Read the model definition and answer for the solid it produces. Units are mm, in the model's axes. A direction names the side the tool comes from. Coordinates: 2 decimals unless noted, no trailing zeros. Order: outer loops, then holes, each group sorted by start corner. A loop starts at its lowest first (then second) coordinate and runs counter-clockwise, first axis right, second up.
from build123d import *

# Parameters (mm, degrees)
SKETCH1_W           = 34
SKETCH1_H           = 29
SKETCH1_R           = 1.4
SKETCH1_R_2         = 1.5
BOSS_EXTRUDE1_DEPTH = 5
BOSS_EXTRUDE2_DEPTH = 5
SKETCH3_R           = 0.85
BOSS_EXTRUDE3_DEPTH = 7
CUT_EXTRUDE2_DEPTH  = 5
FILLET1_R           = 4
SKETCH7_W           = 5
SKETCH7_H           = 34
CUT_EXTRUDE3_DEPTH  = 44
SKETCH8_R           = 1.95
CUT_EXTRUDE4_DEPTH  = 6
FILLET2_R           = 10
BOSS_EXTRUDE4_DEPTH = 4.5
CUT_EXTRUDE5_START  = 4.5
SKETCH9_R           = 2
CUT_EXTRUDE5_DEPTH  = 5
FILLET3_R           = 2


with BuildPart() as part:
    # Sketch1 → Boss-Extrude1 (new body)
    with BuildSketch(Plane.XY):
        with Locations((7.610207842, -10)):
            Rectangle(SKETCH1_W, SKETCH1_H)
        with Locations((15.010207842, 0)):
            Circle(SKETCH1_R, mode=Mode.SUBTRACT)
        with Locations((15.010207842, -20)):
            Circle(SKETCH1_R, mode=Mode.SUBTRACT)
        with Locations((0.010207842, 0)):
            Circle(SKETCH1_R_2, mode=Mode.SUBTRACT)
        with Locations((0.010207842, -20)):
            Circle(SKETCH1_R_2, mode=Mode.SUBTRACT)
    extrude(amount=BOSS_EXTRUDE1_DEPTH)

    # Sketch2 → Boss-Extrude2 (add)
    with BuildSketch(Plane.XZ.offset(24.5)):
        Polygon((-9.389792158, -10), (-9.389792158, 5), (24.610207842, 5), (24.610207842, -48), (14.610207842, -48), align=None)
    extrude(amount=BOSS_EXTRUDE2_DEPTH)

    # Sketch3 → Boss-Extrude3 (add)
    with BuildSketch(Plane(origin=(0, -24.5, 0), x_dir=(1, 0, 0), z_dir=(0, 1, 0))):
        Polygon((24.610207842, 40.5), (9.873365737, 40.5), (13.031260474, 45.5), (24.610207842, 45.5), align=None)
        with Locations(Location((18.031260474, 43, 0), (0, 0, 270))):  # turned: the seam where the file's is
            Circle(SKETCH3_R, mode=Mode.SUBTRACT)
    extrude(amount=BOSS_EXTRUDE3_DEPTH)

    # Sketch6 → Cut-Extrude2 (cut)
    with BuildSketch(Plane(origin=(0, -24.5, 0), x_dir=(1, 0, 0), z_dir=(0, 1, 0))):
        Polygon((13.031260474, 45.5), (24.610207842, 45.5), (24.610207842, 48), (14.610207842, 48), align=None)
    extrude(amount=-CUT_EXTRUDE2_DEPTH, mode=Mode.SUBTRACT)

    # Fillet1
    fillet1_edges = [part.edges().sort_by_distance(p)[0] for p in [
        (17.24178679, -24.5, -40.5),
    ]]
    fillet(fillet1_edges, radius=FILLET1_R)

    # Sketch7 → Cut-Extrude3 (cut)
    with BuildSketch(Plane.ZY.offset(9.389792158)):
        with Locations((2.5, -12.5)):
            Rectangle(SKETCH7_W, SKETCH7_H)
    extrude(amount=-CUT_EXTRUDE3_DEPTH, mode=Mode.SUBTRACT)

    # Sketch8 → Cut-Extrude4 (cut)
    with BuildSketch(Plane.XY):
        with Locations((15.110207842, -27)):
            Circle(SKETCH8_R)
        with Locations(Location((0.110207842, -27, 0), (0, 0, 180))):  # turned: the seam where the file's is
            Circle(SKETCH8_R)
    extrude(amount=-CUT_EXTRUDE4_DEPTH, mode=Mode.SUBTRACT)

    # Fillet2
    fillet2_edges = [part.edges().sort_by_distance(p)[0] for p in [
        (-9.389792158, -27, -10),
    ]]
    fillet(fillet2_edges, radius=FILLET2_R)

    # Sketch11 → Boss-Extrude4 (add)
    with BuildSketch(Plane(origin=(0, -24.5, 0), x_dir=(1, 0, 0), z_dir=(0, 1, 0))):
        with BuildLine():
            Line((1.473365737, 27.2), (4.332633033, 27.2))
            ThreePointArc((4.332633033, 27.2), (5.746846596, 26.614213562), (6.332633033, 25.2))
            Line((6.332633033, 25.2), (6.332633033, 21.2))
            ThreePointArc((6.332633033, 21.2), (5.746846596, 19.785786438), (4.332633033, 19.2))
            Line((4.332633033, 19.2), (-3.579265842, 19.2))
            Line((-3.579265842, 19.2), (1.473365737, 27.2))
        make_face()
    extrude(amount=BOSS_EXTRUDE4_DEPTH)

    # Sketch9 → Cut-Extrude5 (cut)
    with BuildSketch(Plane(origin=(0, -24.5, 0), x_dir=(1, 0, 0), z_dir=(0, 1, 0)).offset(CUT_EXTRUDE5_START)):
        with Locations(Location((2.610207842, 23.2, 0), (0, 0, 90))):  # turned: the seam where the file's is
            Circle(SKETCH9_R)
    extrude(amount=-CUT_EXTRUDE5_DEPTH, mode=Mode.SUBTRACT)

    # Fillet3
    fillet3_edges = [part.edges().sort_by_distance(p)[0] for p in [
        (0.376683596, -24.5, -19.2),
        (5.746846596, -24.5, -19.785786438),
        (6.332633033, -24.5, -23.2),
        (5.746846596, -24.5, -26.614213562),
        (2.902999385, -24.5, -27.2),
    ]]
    fillet(fillet3_edges, radius=FILLET3_R)


solid = part.part
Q1. The part is cut by section A-A, the plane x = 22. Determine the outline of the cut face in (y, z), then the cut area to 3 significant figures.
Q2. Which of the six approach directions +Z, -Z, +X, -X, +Y, -Y give full straight-line access (tool end or side, diameter ignored) to faces 1 (the flat face through (0, -27, -6)), 2 (the flat face through (3, -25, -23)), 3 (the cylindrical face through (6.934, -23.93, -23.172)), 4 (the cylindrical face through (5.73, -21.27, -26.63)), 5 (the flat face through (0, -21, -19.2))?
Q3. The part is cut by section D-D, the plane z = -43. Determine the outline of the cut face in (x, y), then the cut area to 3 significant figures.
Q4. Straight lines are drawn through the part: L1, parallel to X at y = -23.6, z = -23.2; L2, parallel to Y at x = 18, z = -12.5; L3, parallel to X at y = -20.75, z = -43. For each, find the intervals that lie inside material, in ascending order.
Q5. The part is cut by section B-B, the plane y = -26. Determine the outline of the cut face in (x, z).
Q6. The part is cut by section C-C, the plane z = -23.2. Determine the outline of the cut face in (x, y).
Q7. Each of these flat-tipped pins is pushed along its axis until it touches: P1, Ø0.9, axis at x = 15.5, y = -18.5, coming from the +Z side; P2, Ø6, axis at y = -26.5, z = -16, coming from the -X side; P3, Ø3, axis at x = 1, y = -28, coming from the +Z side; P4, Ø4.5, axis at x = 2.5, z = -23.5, coming from the +Y side. Where does it stop, or does it pass through?
Q8. Determine the mould class of faces 6 (the cylindrical face through (14.856, -25.067, -2.958)), 7 (the cylindrical face through (18.07, -21.05, -43.85)), 8 (the cylindrical face through (0.364, -28.933, -2.958)), 9 (the flat face through (12, -29.5, -17)) for opening direction Y: +Y half, -Y half, draft (parallel to the pull), parting line (faces both ways), or undercut.
Computed values:
1. outline: (-29.5, -45.5) - (-17.5, -45.5) - (-17.5, -40.5) - (-20.5, -40.5) arc R4 cw to (-24.5, -36.5) - (-24.5, 0) - (-29.5, 0) - close
1. area: 266 mm2
2. face 1: +Z
2. face 2: +Y
2. face 3: +Z, +X, +Y
2. face 4: -Z, +X, +Y
2. face 5: +Z, +X, -X, +Y
3. outline: (11.45, -29.5) - (24.61, -29.5) - (24.61, -17.5) - (18.88, -17.5) - (18.88, -24.5) - (17.18, -24.5) - (17.18, -17.5) - (11.45, -17.5) - close
3. area: 146 mm2
4. L1: x = -1.05 to 0.61, 4.61 to 6.66
4. L2: y = -29.5 to -24.5
4. L3: x = 11.45 to 17.18, 18.88 to 24.61
5. outline: (-9.39, -7.11) arc R10 ccw to (-7.84, -12.45) - (13.03, -45.5) - (24.61, -45.5) - (24.61, 0) - (16.78, 0) - (16.78, -6) - (13.44, -6) - (13.44, 0) - (1.78, 0) - (1.78, -6) - (-1.56, -6) - (-1.56, 0) - (-9.39, 0) - close
6. outline: (-1.05, -29.5) - (24.61, -29.5) - (24.61, -24.5) - (8.33, -24.5) arc R2 cw to (6.33, -22.5) - (6.33, -20) - (4.61, -20) - (4.61, -25) - (0.61, -25) - (0.61, -20) - (-1.05, -20) - close
7. P1: stops at z = -40.5
7. P2: stops at x = -7.5
7. P3: stops at z = 0
7. P4: stops at y = -20
8. face 6: undercut
8. face 7: draft
8. face 8: undercut
8. face 9: -Y half
